Can you work these out from the model? Positions are in its coordinate system, mm. A direction names the side the tool comes from. Round coordinates to 2 decimals unless told otherwise and drop trailing zeros. Loops run counter-clockwise (first coordinate to the right, second up) from the corner with the lowest first, then second, coordinate; pieces in that order, holes last. Notation, with made-up numbers: (78, 54.25) -> (84, 54.25) arc R9 ccw to (84, 67.25) -> close; hole circle Ø9 at (-2, -11). An arc over 180 degrees is marked (long way). Write item = value, one per line.
from build123d import *

# Parameters (mm, degrees)
F1_DEPTH = 63.5
F0_W     = 25.4
F0_H     = 19.05
F2_DEPTH = 12.7
F3_DEPTH = 7.9375


with BuildPart() as f1:
    # F0 (on Front) → F1 (new body, symmetric)
    with BuildSketch(Plane.XZ):
        Polygon((41.275, -9.525), (41.275, 9.525), (22.225, 9.525), (-41.275, 9.525), (-41.275, -9.525), align=None)
    extrude(amount=F1_DEPTH, both=True)

    # F0 (on Front) → F2 (join, symmetric)
    with BuildSketch(Plane.XZ):
        with BuildLine():
            Line((22.225, 9.525), (41.275, 9.525))
            Line((41.275, 9.525), (41.275, 27.0002))
            ThreePointArc((41.275, 27.0002), (45.9246798487, 38.2255201513), (57.15, 42.8752))
            Line((57.15, 42.8752), (60.325, 42.8752))
            Line((60.325, 42.8752), (60.325, 61.9252))
            Line((60.325, 61.9252), (57.15, 61.9252))
            add(Edge.make_bspline(
                [(57.15, 61.9252), (57.0373941286, 61.9247746009), (56.9247198361, 61.9242293137), (56.8119782106, 61.9235641889)],
                knots=[0, 0, 0, 0, 0.2853238396, 0.2853238396, 0.2853238396, 0.2853238396], degree=3))
            ThreePointArc((56.8119782106, 61.9235641889), (32.3350746929, 51.5761050088), (22.225, 27.0002))
            Line((22.225, 27.0002), (22.225, 9.525))
        make_face()
        with Locations((73.025, 52.4002)):
            Rectangle(F0_W, F0_H)
    extrude(amount=F2_DEPTH, both=True)

    # F0 (on Front) → F3 (join, symmetric)
    with BuildSketch(Plane.XZ):
        with BuildLine():
            Line((-41.275, 9.525), (22.225, 9.525))
            Line((22.225, 9.525), (22.225, 27.0002))
            ThreePointArc((22.225, 27.0002), (32.3350746929, 51.5761050088), (56.8119782106, 61.9235641889))
            add(Edge.make_bspline(
                [(56.8119782106, 61.9235641889), (12.8653006287, 61.6642986017), (-41.3122228032, 43.1964478653), (-41.275, 9.525)],
                knots=[0.2853238396, 0.2853238396, 0.2853238396, 0.2853238396, 111.5045361635, 111.5045361635, 111.5045361635, 111.5045361635], degree=3))
        make_face()
    extrude(amount=F3_DEPTH, both=True)

    # F0 (on Front) → F4 (revolve)
    with BuildSketch(Plane.XZ):
        Polygon((85.725, 61.9252), (85.725, 42.8752), (85.725, 38.1), (111.125, 38.1), (111.125, 66.675), (85.725, 66.675), align=None)
    revolve(axis=Axis((85.725, 0, 52.3875), (0, 0, -1)))


solid = f1.part
1. Suppose I cut it at A-A, the plane y = -14.5. List the corners of the cut face in (x, z) for me (1 decimal).
Entries:
outline = (-41.3, -9.5) -> (41.3, -9.5) -> (41.3, 9.5) -> (-41.3, 9.5) -> close; (64.9, 38.1) -> (106.6, 38.1) -> (106.6, 66.7) -> (64.9, 66.7) -> close
2. Suppose I cut it at C-C, the plane y = 20. List the corners of the cut face in (x, z) for me (3 decimals), and give its area (3 significant figures).
Entries:
outline = (-41.275, -9.525) -> (41.275, -9.525) -> (41.275, 9.525) -> (-41.275, 9.525) -> close; (70.067, 38.1) -> (101.383, 38.1) -> (101.383, 66.675) -> (70.067, 66.675) -> close
area = 2,470 mm²
3. Suppose I cut it at B-B, the plane y = -32. List the corners of the cut face in (x, z) for me (3 decimals), and give its area (3 significant figures).
Entries:
outline = (-41.275, -9.525) -> (41.275, -9.525) -> (41.275, 9.525) -> (-41.275, 9.525) -> close
area = 1,570 mm²
4. We'd pull the mould along X, two halves only. Please class faces 6 (the cylindrical face through (45.8, -0.2, 38.1)), 7 (the cylindrical face through (32.61, 10.29, 51.85)), 8 (the flat face through (85, 0, 66.675)): released by +X, released by -X, zero draft, split by the parting line, or undercut.
Entries:
face_6 = undercut
face_7 = released by -X
face_8 = zero draft
5. I need wall thicknesses on line 1 (Z direction, x = -3, y = 55.5) (3 decimals); line 2 (Z direction, x = 103, y = -0.5) (3 decimals); line 3 (X direction, y = -20, z = 7) (3 decimals). Which ranges of each line are inside material? Lowest first, please. Write a range as [from, to].
Entries:
line_1 = [-9.525, 9.525]
line_2 = [38.1, 66.675]
line_3 = [-41.275, 41.275]
6. I'm going to push flat-ended pins straight in: pin 1 (4 mm diameter, centred on x = 20, y = 20.5, fed in from +Z) (3 decimals); pin 2 (2 mm diameter, centred on x = 60.5, y = 1, fed in from -Z); pin 3 (10 mm diameter, centred on x = 10, z = 50.5, fed in from -Y); pin 4 (12.5 mm diameter, centred on x = 53, z = 29, fed in from -Y). Where does each tip first touch, or does it pass through?
Entries:
pin_1 = 9.525
pin_2 = 38.1
pin_3 = -7.94
pin_4 = through
7. For faces 1 (the flat face through (38, -12.7, 36)), 2 (the flat face through (41.275, -1, 0)), 3 (the flat face through (38, 12.7, 36)), 4 (the flat face through (60, 0, 61.925)), 5 (the flat face through (60, 0, 42.875)), which set-ups out of +Z, -Z, +X, -X, +Y, -Y let a thin tool reach every point of the face, with its end or its side?
Entries:
face_1 = +Z, -X, -Y
face_2 = -Z, +X, +Y, -Y
face_3 = +Z, -X, +Y
face_4 = +Z, -X
face_5 = -Z
8. Suppose I cut it at D-D, the plane x = 74. List the corners of the cut face in (y, z) for me (3 decimals), and give its area (3 significant figures).
Entries:
outline = (-22.532, 38.1) -> (22.532, 38.1) -> (22.532, 66.675) -> (-22.532, 66.675) -> close
area = 1,290 mm²
